```python
from build123d import *

# Parameters (mm, degrees)
SKETCH1_R           = 1.5
BOSS_EXTRUDE1_DEPTH = 3
CUT_EXTRUDE2_DEPTH  = 0.9
SKETCH5_W           = 3.6
SKETCH5_H           = 3
FILLET1_R           = 2.5


with BuildPart() as part:
    # Sketch1 → Boss-Extrude1 (new body)
    with BuildSketch(Plane.XY.offset(1.9)):
        with BuildLine():
            Line((2.5, -11), (2.5, -4.330127019))
            ThreePointArc((2.5, -4.330127019), (5, 0), (2.5, 4.330127019))
            Line((2.5, 4.330127019), (2.5, 55))
            ThreePointArc((2.5, 55), (0, 57.5), (-2.5, 55))
            Line((-2.5, 55), (-2.5, 8.124038405))
            ThreePointArc((-2.5, 8.124038405), (-2.735010245, 8.047963653), (-2.967710696, 7.965092167))
            Line((-2.967710696, 7.965092167), (-3.054167872, 8.093270203))
            ThreePointArc((-3.054167872, 8.093270203), (-4.342095244, 9.472160372), (-5.994566265, 10.382893341))
            ThreePointArc((-5.994566265, 10.382893341), (-6.032083889, 8.496444973), (-5.481893659, 6.691622066))
            Line((-5.481893659, 6.691622066), (-5.414116812, 6.552658937))
            ThreePointArc((-5.414116812, 6.552658937), (-6.01040764, 6.01040764), (-6.552658937, 5.414116812))
            Line((-6.552658937, 5.414116812), (-6.691622066, 5.481893659))
            ThreePointArc((-6.691622066, 5.481893659), (-8.496444973, 6.032083889), (-10.382893341, 5.994566265))
            ThreePointArc((-10.382893341, 5.994566265), (-9.472160372, 4.342095244), (-8.093270203, 3.054167872))
            Line((-8.093270203, 3.054167872), (-7.965092167, 2.967710696))
            ThreePointArc((-7.965092167, 2.967710696), (-8.210369523, 2.199961883), (-8.381827508, 1.41243323))
            Line((-8.381827508, 1.41243323), (-8.536061531, 1.401648136))
            ThreePointArc((-8.536061531, 1.401648136), (-10.374179133, 0.975715399), (-11.989132531, 0))
            ThreePointArc((-11.989132531, 0), (-10.374179133, -0.975715399), (-8.536061531, -1.401648136))
            Line((-8.536061531, -1.401648136), (-8.381827508, -1.41243323))
            ThreePointArc((-8.381827508, -1.41243323), (-8.210369523, -2.199961883), (-7.965092167, -2.967710696))
            Line((-7.965092167, -2.967710696), (-8.093270203, -3.054167872))
            ThreePointArc((-8.093270203, -3.054167872), (-9.472160372, -4.342095244), (-10.382893341, -5.994566265))
            ThreePointArc((-10.382893341, -5.994566265), (-8.496444973, -6.032083889), (-6.691622066, -5.481893659))
            Line((-6.691622066, -5.481893659), (-6.552658937, -5.414116812))
            ThreePointArc((-6.552658937, -5.414116812), (-6.01040764, -6.01040764), (-5.414116812, -6.552658937))
            Line((-5.414116812, -6.552658937), (-5.481893659, -6.691622066))
            ThreePointArc((-5.481893659, -6.691622066), (-6.032083889, -8.496444973), (-5.994566265, -10.382893341))
            ThreePointArc((-5.994566265, -10.382893341), (-4.342095244, -9.472160372), (-3.054167872, -8.093270203))
            Line((-3.054167872, -8.093270203), (-2.967710696, -7.965092167))
            ThreePointArc((-2.967710696, -7.965092167), (-2.735010245, -8.047963653), (-2.5, -8.124038405))
            Line((-2.5, -8.124038405), (-2.5, -11))
            Line((-2.5, -11), (2.5, -11))
        make_face()
        with Locations((0, 55)):
            Circle(SKETCH1_R, mode=Mode.SUBTRACT)
    extrude(amount=-BOSS_EXTRUDE1_DEPTH)

    # Sketch4 → Cut-Extrude2 (cut)
    with BuildSketch(Plane.XY.offset(1.9)):
        with BuildLine():
            Line((-5.102940329, -2.6), (-1.358771093, -3.333727811))
            ThreePointArc((-1.358771093, -3.333727811), (-3.6, 0), (-1.358771093, 3.333727811))
            Line((-1.358771093, 3.333727811), (-5.102940329, 2.6))
            Line((-5.102940329, 2.6), (-5.102940329, -2.6))
        make_face()
    extrude(amount=-CUT_EXTRUDE2_DEPTH, mode=Mode.SUBTRACT)

    # Sketch5 → Cut-Revolve1 (revolve, cut)
    with BuildSketch(Plane(origin=(0, 0, 0), x_dir=(1, 0, 0), z_dir=(0, 1, 0))):
        with Locations((1.8, -1.5)):
            Rectangle(SKETCH5_W, SKETCH5_H)
    revolve(axis=Axis((0, 0, 0), (0, 0, 1)), mode=Mode.SUBTRACT)

    # Chamfer1
    # the kernel refuses this chamfer: 1.996823512, 1.412365401 mm, written as the material it takes off along each edge
    with BuildSketch(Plane(origin=(-5.994566265, -10.382893341, 6.307600342), x_dir=(0.8971018613245074, 0.44182377754949315, 0), z_dir=(0, 0, -1)), Plane(origin=(-10.382893341, -5.994566265, 6.307600342), x_dir=(0.9978248904640776, -0.06592031530834441, 0), z_dir=(0, 0, -1)), Plane(origin=(-11.989132531, 0, 6.307600342), x_dir=(0.8311815460161414, -0.5560011129145489, 0), z_dir=(0, 0, -1))) as chamfer1_piece_1:
        with BuildLine():
            Line((1.33889649, 0), (0.700148491, -1.556942978))
            ThreePointArc((0.700148491, -1.556942978), (0.305807457, -0.828670891), (0, 0))
            ThreePointArc((0, 0), (0.684607685, 0.037444556), (1.33889649, 0))
        make_face()
    extrude(amount=11.815200684, mode=Mode.SUBTRACT)
    with BuildSketch(Plane(origin=(-10.382893341, 5.994566265, 6.307600342), x_dir=(0.9993864811320993, 0.035023725250178994, 0), z_dir=(0, 0, -1)), Plane(origin=(-5.994566265, 10.382893341, 6.307600342), x_dir=(0.883005943484212, -0.4693618047642527, 0), z_dir=(0, 0, -1))) as chamfer1_piece_2:
        with BuildLine():
            Line((1.707126049, 0), (0.549125448, 1.221108125))
            ThreePointArc((0.549125448, 1.221108125), (0.246629708, 0.639737105), (0, 0))
            ThreePointArc((0, 0), (0.881190909, -0.060960877), (1.707126049, 0))
        make_face()
    extrude(amount=11.815200684, mode=Mode.SUBTRACT)

    # Fillet1
    fillet1_edges = [part.edges().sort_by_distance(p)[0] for p in [
        (2.5, -11, 0.4),
    ]]
    fillet(fillet1_edges, radius=FILLET1_R)


solid = part.part
```
Part model, mm, in its own coordinate system. A direction names the side the tool comes from. Give positions to 0.01 mm unless a question says otherwise; leave off trailing zeros. Write each loop counter-clockwise with the first axis right and the second up, starting at its lowest first coordinate (ties: lowest second). Pieces come first, ordered by that corner, then holes. Notation, with made-up numbers: (74, -5.75) -> (113, -5.75) arc R23 cw to (113, 3.25) -> close; hole circle Ø11 at (33.5, 45). An arc over 180 degrees is marked (long way). Put each result on its own line as item: value. Start each with the question number.
Item 1: Wall check: L1, parallel to Y at x = -1, z = 0.4; L2, parallel to Y at x = 0.5, z = 0.3; L3, parallel to X at y = 26.5, z = 0.75. Give the ranges that are in metal, low to high. Write a range as [from, to].
Item 2: Cut at A-A (y = 0). List the corners of the cut face in (x, z), then the cut area to 3 significant figures.
Item 3: Pull direction X, two halves, no side cores. Call faces 4 (the face through (-9.756, -1.188, 0.421)), 5 (the face through (-1, 16, 1.9)), 6 (the face through (-1.2, 54.1, 0.4)): pulls with the +X half, pulls with the -X half, needs draft (parallel to the pull), parting line crosses it, or undercut.
Item 4: Cut at B-B (y = 43). List the corners of the cut face in (x, z), then the cut area to 3 significant figures.
Item 5: Which spindle directions (+Z, -Z, +X, -X, +Y, -Y) get a long thin tool onto all of the face, cutting with end or side? Do faces 1 (the face through (-4, 0, 1)), 2 (the face through (2.5, 29, 0)), 3 (the face through (-8.889, -3.696, 0.421)). Say none if no direction does.
Item 6: Pin check, flat tips, straight feed: pin 1 Ø1 at (x, y) = (-8.5, -3) entering from +Z; pin 2 Ø1.4 at (y, z) = (-10, 0.5) entering from -X; pin 3 Ø0.9 at (y, z) = (-5.5, 0.5) entering from +X; pin 4 Ø3.5 at (x, y) = (0, -1.5) entering from +Z. Stop position of each tip, or through.
Answer list:
1. L1: y = [-11, -3.46], [3.46, 53.88], [56.12, 57.29]
1. L2: y = [-10.95, -3.57], [3.57, 53.59], [56.41, 57.45]
1. L3: x = [-2.5, 2.5]
2. outline: (-10.73, -1.1) -> (5, -1.1) -> (5, 1.9) -> (3.6, 1.9) -> (3.6, 0) -> (-3.6, 0) -> (-3.6, 1) -> (-5.1, 1) -> (-5.1, 1.9) -> (-10.73, 1.9) -> close
2. area: 32.1 mm2
3. face 4: pulls with the -X half
3. face 5: needs draft
3. face 6: undercut
4. outline: (-2.5, -1.1) -> (2.5, -1.1) -> (2.5, 1.9) -> (-2.5, 1.9) -> close
4. area: 15.0 mm2
5. face 1: +Z
5. face 2: +Z, -Z, +X, +Y
5. face 3: +Z, -Z, -X
6. pin 1: stops at z = 1.9
6. pin 2: stops at x = -5.35
6. pin 3: stops at x = 2.5
6. pin 4: stops at z = 0
